from build123d import *

# Parameters (mm, degrees)
SKETCH_1_R          = 21.15
EXTRUDE_1_DEPTH     = 10
SKETCH_2_R          = 1.6
CUT_EXTRUDE_1_DEPTH = 64.50267784
CUT_EXTRUDE_START   = -5
SKETCH_3_R          = 2.9
CUT_EXTRUDE_2_DEPTH = 59.502677944
CUT_EXTRUDE_5_DEPTH = 43.187291864


with BuildPart() as part:
    # 草图1 → 凸台-拉伸1 (new body)
    with BuildSketch(Plane.XY):
        with BuildLine():
            Line((-27.924319022, -30), (27.075680978, -30))
            Line((27.075680978, -30), (26.137883686, 0.795950004))
            ThreePointArc((26.137883686, 0.795950004), (0.355472008, 26.147583821), (-26.106586279, 1.506204794))
            Line((-26.106586279, 1.506204794), (-27.924319022, -30))
        make_face()
        Circle(SKETCH_1_R, mode=Mode.SUBTRACT)
    extrude(amount=EXTRUDE_1_DEPTH)

    # 草图2 → 切除-拉伸1 (cut, through all)
    with BuildSketch(Plane.XZ.offset(30)):
        with Locations(Location((10.425680978, 5, 0), (0, 0, 270))):
            Circle(SKETCH_2_R)
        with Locations(Location((-9.574319022, 5, 0), (0, 0, 270))):
            Circle(SKETCH_2_R)
    extrude(amount=-CUT_EXTRUDE_1_DEPTH, mode=Mode.SUBTRACT)

    # 草图3 → 切除-拉伸2 (cut, through all)
    with BuildSketch(Plane.XZ.offset(30).offset(CUT_EXTRUDE_START)):
        with Locations(Location((10.425680978, 5, 0), (0, 0, 270))):
            Circle(SKETCH_3_R)
        with Locations(Location((-9.574319022, 5, 0), (0, 0, 270))):
            Circle(SKETCH_3_R)
    extrude(amount=-CUT_EXTRUDE_2_DEPTH, mode=Mode.SUBTRACT)

    # 草图4 → 切除-拉伸5 (cut, through all)
    with BuildSketch(Plane(origin=(0, 0, 0), x_dir=(-1, 0, 0), z_dir=(0, 0, -1))):
        with BuildLine():
            Line((-7.858993685, 25.04593217), (21.750509975, 14.696183717))
            ThreePointArc((21.750509975, 14.696183717), (8.661574884, 24.779822851), (-7.858993685, 25.04593217))
        make_face()
    extrude(amount=-CUT_EXTRUDE_5_DEPTH, mode=Mode.SUBTRACT)


solid = part.part
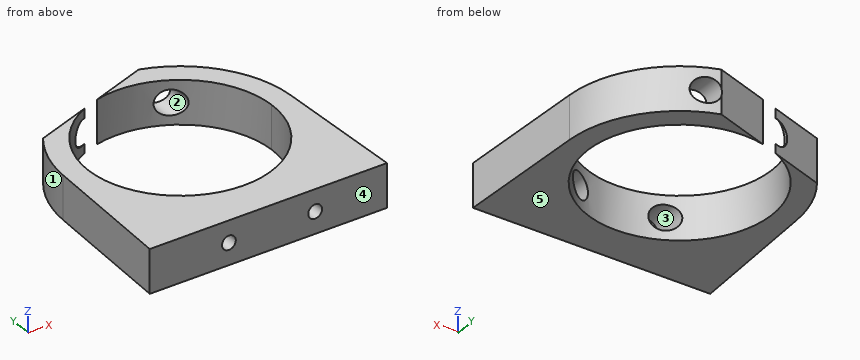
For this review, take the finished solid that the model builds, in its own axes (mm). Face numbers are marked on the shaded views. A direction names the side the tool comes from. Round coordinates to 2 decimals unless told otherwise and drop trailing zeros. Order: outer loops, then holes, each group sorted by start corner. A loop starts at its lowest first (then second) coordinate and runs counter-clockwise, first axis right, second up. Notation, with made-up numbers: M -21.5,-25 L 9.5,-25 A26 cw 9.5,14 Z; hole C 2.25,-26 d10. An arc over 180 degrees is marked long. Use a Markdown table: item, result. Add a question column.
Item 1: Mouldability with a two-part tool opening along Z and no side actions: class the marked faces 3, 4 and 5 as released by +Z, released by -Z, zero draft, split by the parting line, or undercut.
Item 2: Tool access review of the marked faces 1 and 2: name each direction out of +Z, -Z, +X, -X, +Y, -Y from which nothing blocks a thin tool from reaching the whole face with its end or side.
Item 3: Insertion check: pin 1 (1.7 mm diameter, centred on x = 10, z = 6, fed in from +Y); pin 2 (1 mm diameter, centred on y = -10.5, z = 3, fed in from +X); pin 3 (6 mm diameter, centred on y = 2, z = 2, fed in from -X). Each pin has a flat end and moves straight along its axis. Give the tip position at first contact, or say it passes through.
Item 4: To check wall thickness, follow line 1 along X through (y, z) = (-26.6, 5); line 2 along Y through (x, z) = (-10.5, 7.25); line 3 along X through (y, z) = (-22.5, 5). State the ranges of each line that lie inside material, in increasing order.
Item 5: Add section B-B, the plane z = 5. Give the boundary of the cut face in (x, y).
Item 6: Add section D-D, the plane y = 9. Give the boundary of the cut face in (x, z), then the cut area to 3 significant figures.
Item 7: Add section A-A, the plane y = -20. Give the boundary of the cut face in (x, z).
Item 8: Add section C-C, the plane x = -18. Give the boundary of the cut face in (y, z).
Geometry results:
| question | item | result |
|---|---|---|
| 1 | face 3 | undercut |
| 1 | face 4 | zero draft |
| 1 | face 5 | released by -Z |
| 2 | face 1 | +Z, -Z, -X, +Y |
| 2 | face 2 | +Y |
| 3 | pin 1 | stops at y = -25 |
| 3 | pin 2 | stops at x = 26.5 |
| 3 | pin 3 | stops at x = -26.25 |
| 4 | line 1 | x = -27.73 to -11.17, -7.97 to 8.83, 12.03 to 26.97 |
| 4 | line 2 | y = -30 to -25 |
| 4 | line 3 | x = -27.49 to -12.47, -6.67 to 7.53, 13.33 to 26.85 |
| 5 | outline | M -27.92,-30 L -11.17,-30 L -11.17,-25 L -12.47,-25 L -12.47,-17.08 A21.15 cw -12.47,17.08 L -12.47,17.94 L -21.59,14.75 A26.15 ccw -26.11,1.51 Z; M -7.97,-30 L 8.83,-30 L 8.83,-25 L 7.53,-25 L 7.53,-19.77 A21.15 cw -6.67,-20.07 L -6.67,-25 L -7.97,-25 Z; M -5.01,20.55 A21.15 cw 7.53,19.77 L 7.53,24.93 Z; M 12.03,-30 L 27.08,-30 L 26.14,0.8 A26.15 ccw 13.33,22.5 L 13.33,16.42 A21.15 cw 13.33,-16.42 L 13.33,-25 L 12.03,-25 Z |
| 6 | outline | M -24.55,0 L -19.14,0 L -19.14,10 L -24.55,10 Z; M 19.14,0 L 24.55,0 L 24.55,10 L 19.14,10 Z |
| 6 | area | 108 mm² |
| 7 | outline | M -27.35,0 L -6.88,0 L -6.88,3.93 A2.9 cw long -6.88,6.07 L -6.88,10 L -27.35,10 Z; M 6.88,0 L 26.77,0 L 26.77,10 L 6.88,10 Z; hole C 10.43,5 d5.8 |
| 8 | outline | M -30,0 L -11.11,0 L -11.11,10 L -30,10 Z; M 11.11,0 L 16.01,0 L 16.01,10 L 11.11,10 Z |
